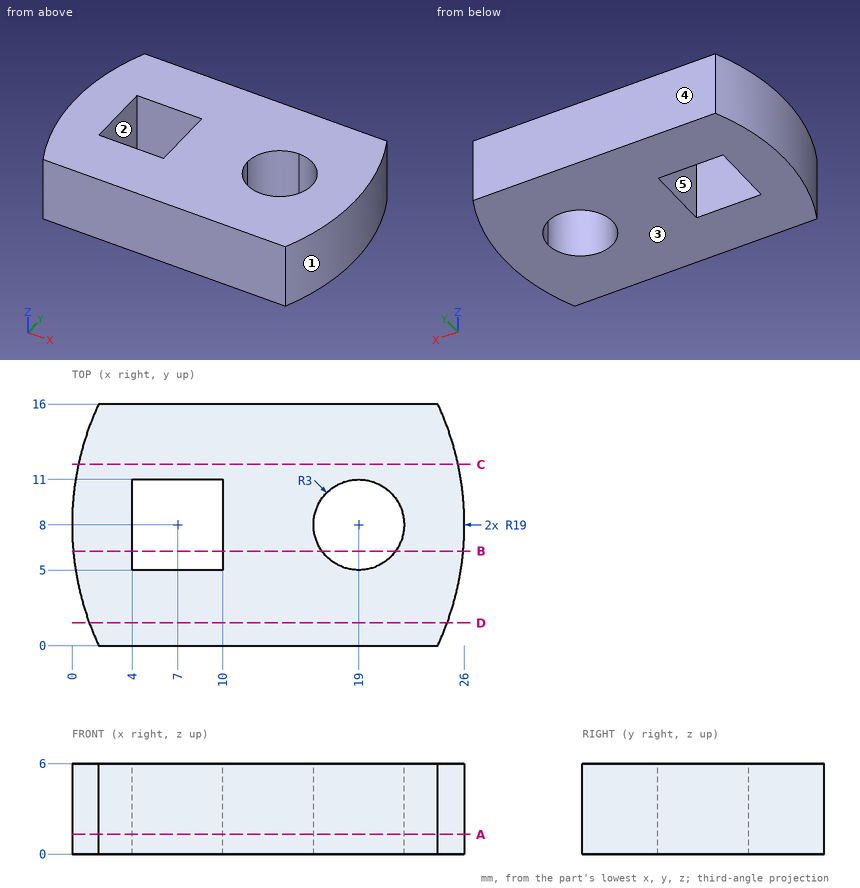
Print and shaded views of the part. All mm, measured from the part's lowest x, y and z. A direction names the side the tool comes from. Coordinates: 2 decimals unless noted, no trailing zeros. Order: outer loops, then holes, each group sorted by start corner. A loop starts at its lowest first (then second) coordinate and runs counter-clockwise, first axis right, second up. Notation, with made-up numbers: M -32,13 L -27,13 A14 ccw -27,19 Z; hole C -36,-10.5 d6. An arc over 180 degrees is marked long. One line per question, with ' | ' between items. Start each with the question number.
Q1. Two-plate mould, pull along X, no slides. Class the marked faces 1, 2 and 3: +X half, -X half, draft (parallel to the pull), parting line (faces both ways), or undercut.
Q2. Saw through at A-A (z = 1.3). List the corners of the cut face in (x, y), then the cut area to 3 significant figures.
Q3. 3-axis set-ups, long thin cutter, end or side, ignore diameter. For the marked faces 4 and 5: which of +Z, -Z, +X, -X, +Y, -Y reach the whole face in a straight line?
Q4. Saw through at C-C (y = 12). List the corners of the cut face in (x, z).
Q5. Flat gauge pins, fed straight in: pin 1 Ø2 at (y, z) = (11, 2) entering from -X; pin 2 Ø3 at (y, z) = (8, 2.5) entering from -X; pin 3 Ø3 at (y, z) = (7, 2.5) entering from +X. Where does each tip first touch, or does it go through?
Q6. Saw through at B-B (y = 6.25). List the corners of the cut face in (x, z).
Q7. Probe L1, parallel to X at y = 9.5, z = 3.35; L2, parallel to X at y = 10.5, z = 4.05; L3, parallel to Y at x = 5.75, z = 0.45. List the from-to ranges inside material, lowest first. Write a range as from..to.
Q8. Saw through at D-D (y = 1.5). List the corners of the cut face in (x, z).
Check values:
1) face 1: +X half | face 2: undercut | face 3: draft
2) outline: M 1.77,0 L 24.23,0 A19 ccw 24.23,16 L 1.77,16 A19 ccw Z; hole M 4,5 L 10,5 L 10,11 L 4,11 Z; hole M 16,8 A3 ccw 22,8 A3 ccw 19,11 A3 ccw Z | area: 333 mm2
3) face 4: +Z, -Z, +X, -X, +Y | face 5: +Z, -Z
4) outline: M 0.43,0 L 25.57,0 L 25.57,6 L 0.43,6 Z
5) pin 1: stops at x = 0.11 | pin 2: stops at x = 0 | pin 3: stops at x = 26
6) outline: M 0.08,0 L 4,0 L 4,6 L 0.08,6 Z; M 10,0 L 16.56,0 L 16.56,6 L 10,6 Z; M 21.44,0 L 25.92,0 L 25.92,6 L 21.44,6 Z
7) L1: x = 0.06..4, 10..16.4, 21.6..25.94 | L2: x = 0.17..4, 10..17.34, 20.66..25.83 | L3: y = 0..5, 11..16
8) outline: M 1.15,0 L 24.85,0 L 24.85,6 L 1.15,6 Z
